Input: part model. Units: mm. Frame: model coordinates. Face numbers are marked on the shaded views. A direction names the side the tool comes from. Give positions to 0.01 mm unless a question says otherwise; leave off trailing zeros. Loops run counter-clockwise (first coordinate to the right, second up) from the corner with the lowest first, then second, coordinate; pieces in that order, holes last. Notation, with made-up numbers: (3, -28.75) -> (54, -28.75) arc R4 ccw to (54, -22.75) -> close; hole circle Ø1 at (79, 73.25). An arc over 180 degrees is marked (long way). Answer in a Markdown table with one row per item. Add a question column.
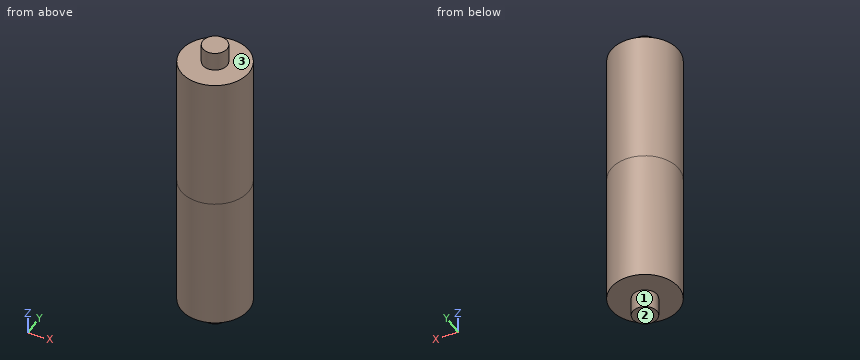
```python
from build123d import *

# Parameters (mm, degrees)
SKETCH2_R           = 4.5
BOSS_EXTRUDE1_DEPTH = 7
SKETCH3_R           = 12.5
BOSS_EXTRUDE2_DEPTH = 50


with BuildPart() as part:
    # Sketch2 → Boss-Extrude1 (new body)
    with BuildSketch(Plane.XY):
        Circle(SKETCH2_R)
    extrude(amount=BOSS_EXTRUDE1_DEPTH)

    # Sketch3 → Boss-Extrude2 (add)
    with BuildSketch(Plane.XY.offset(7)):
        Circle(SKETCH3_R)
    extrude(amount=BOSS_EXTRUDE2_DEPTH)

    # Mirror1: part across plane


with BuildPart() as part_1:
    add(part.part)
    add(part.part.mirror(Plane.XY.offset(57)))


solid = part_1.part
```
1) Section D-D on y = 7.5. Output: boundary loops of the cut face in (x, z), and give its area (3 significant figures).
2) Reachability of the marked faces 1, 2 and 3 from +Z, -Z, +X, -X, +Y, -Y: full face, straight path, thin tool, end or side. Return the list, or none.
3) Section A-A on y = 0. Output: boundary loops of the cut face in (x, z).
4) Material intervals for line 1 along Y through (x, z) = (0.5, 57); line 2 along Z through (x, y) = (-11.5, -2); line 3 along Y through (x, z) = (8, 47), sorted ascending.
5) Pin query (flat end, axial travel): pin 1 (1.5 mm diameter, centred on y = 8.5, z = 41.5, fed in from +X); pin 2 (2 mm diameter, centred on y = 5, z = 84.5, fed in from +X); pin 3 (1 mm diameter, centred on x = -7, z = 69.5, fed in from +Y). Return the tip coordinate at first contact, or that it passes through.
6) Section C-C on z = 58. Output: boundary loops of the cut face in (x, y), and give its area (3 significant figures).
Working result:
| question | item | result |
|---|---|---|
| 1 | outline | (-10, 7) -> (10, 7) -> (10, 107) -> (-10, 107) -> close |
| 1 | area | 2,000 mm2 |
| 2 | face 1 | -Z |
| 2 | face 2 | -Z, +X, -X, +Y, -Y |
| 2 | face 3 | +Z |
| 3 | outline | (-12.5, 7) -> (-4.5, 7) -> (-4.5, 0) -> (4.5, 0) -> (4.5, 7) -> (12.5, 7) -> (12.5, 107) -> (4.5, 107) -> (4.5, 114) -> (-4.5, 114) -> (-4.5, 107) -> (-12.5, 107) -> close |
| 4 | line 1 | y = -12.49 to 12.49 |
| 4 | line 2 | z = 7 to 107 |
| 4 | line 3 | y = -9.6 to 9.6 |
| 5 | pin 1 | stops at x = 9.81 |
| 5 | pin 2 | stops at x = 11.84 |
| 5 | pin 3 | stops at y = 10.68 |
| 6 | outline | circle Ø25 at (0, 0) |
| 6 | area | 491 mm2 |
